CAD build for the part. Positions are in the model's coordinates, mm. Face numbers are marked on the shaded views. A direction names the side the tool comes from. Coordinates: 2 decimals unless noted, no trailing zeros. Loops run counter-clockwise (first coordinate to the right, second up) from the corner with the lowest first, then second, coordinate; pieces in that order, holes last.
1) Saw through at B-B, the plane x = 0. Write the cut outline in (y, z) (1 decimal), and give its area (3 significant figures).
2) Saw through at C-C, the plane z = 0. Write the cut outline in (x, y) (1 decimal), and give its area (3 significant figures).
3) Saw through at A-A, the plane y = -8.5. Write the cut outline in (x, z) (3 decimals), and give its area (3 significant figures).
4) Which spindle directions (+Z, -Z, +X, -X, +Y, -Y) get a long thin tool onto all of the face, cutting with end or side? Do the marked faces 4, 5 and 6. Say none if no direction does.
5) Saw through at D-D, the plane y = -16. Write the cut outline in (x, z), and give its area (3 significant figures).
6) Wall check: line 1 along Z through (x, y) = (0, -12) (3 decimals); line 2 along Z through (x, y) = (2, -12.25); line 3 along X through (y, z) = (-10.25, 2.75). Give the ranges that are in metal, low to high.
7) Pin check, flat tips, straight feed: pin 1 Ø8 at (x, y) = (5.5, -5.5) entering from +Z; pin 2 Ø1 at (y, z) = (-11.5, -4) entering from +X; pin 3 Ø3 at (x, z) = (6.5, 2) entering from -Y; pin 4 Ø9.5 at (x, z) = (-3, 2) entering from -Y. Stop position of each tip, or through.
8) Two-plate mould, pull along Z, no slides. Class the marked faces 1, 2 and 3: +Z half, -Z half, draft (parallel to the pull), parting line (faces both ways), or undercut.
```python
from build123d import *

# Parameters (mm, degrees)
F0_R     = 9.525
F1_DEPTH = 14.2875
F2_R     = 8.150668
F3_DEPTH = 1.5875
F4_R     = 7.451833
F5_DEPTH = 6.35
F6_R     = 3
F7_DEPTH = 9.525


with BuildPart() as f1:
    # F0 (on Front) → F1 (new body)
    with BuildSketch(Plane.XZ):
        Circle(F0_R)
    extrude(amount=F1_DEPTH)

    # F2 (on face) → F3 (join)
    with BuildSketch(Plane(origin=(0, 0, 0), x_dir=(-1, 0, 0), z_dir=(0, 1, 0))):
        Circle(F2_R)
    extrude(amount=F3_DEPTH)

    # F4 (on face) → F5 (cut)
    with BuildSketch(Plane.XZ.offset(14.2875)):
        Circle(F4_R)
    extrude(amount=-F5_DEPTH, mode=Mode.SUBTRACT)

    # F6 (on face) → F7 (join)
    with BuildSketch(Plane.XZ.offset(7.9375)):
        Circle(F6_R)
    extrude(amount=F7_DEPTH)


solid = f1.part
```
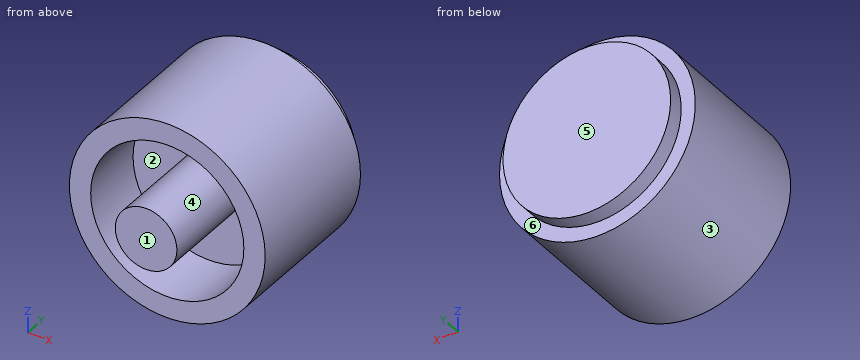
Data:
1. outline: (-17.5, -3) - (-7.9, -3) - (-7.9, -7.5) - (-14.3, -7.5) - (-14.3, -9.5) - (0, -9.5) - (0, -8.2) - (1.6, -8.2) - (1.6, 8.2) - (0, 8.2) - (0, 9.5) - (-14.3, 9.5) - (-14.3, 7.5) - (-7.9, 7.5) - (-7.9, 3) - (-17.5, 3) - close
1. area: 261 mm2
2. outline: (-9.5, -14.3) - (-7.5, -14.3) - (-7.5, -7.9) - (-3, -7.9) - (-3, -17.5) - (3, -17.5) - (3, -7.9) - (7.5, -7.9) - (7.5, -14.3) - (9.5, -14.3) - (9.5, 0) - (8.2, 0) - (8.2, 1.6) - (-8.2, 1.6) - (-8.2, 0) - (-9.5, 0) - close
2. area: 261 mm2
3. outline: circle Ø19.05 at (0, 0); circle Ø6 at (0, 0); hole circle Ø14.904 at (0, 0)
3. area: 139 mm2
4. face 4: -Y
4. face 5: +Z, -Z, +X, -X, +Y
4. face 6: +Y
5. outline: circle Ø6 at (0, 0)
5. area: 28.3 mm2
6. line 1: z = -9.525 to -7.452, -3 to 3, 7.452 to 9.525
6. line 2: z = -9.31 to -7.18, -2.24 to 2.24, 7.18 to 9.31
6. line 3: x = -9.12 to -6.93, -1.2 to 1.2, 6.93 to 9.12
7. pin 1: stops at z = 9.41
7. pin 2: stops at x = 8.86
7. pin 3: stops at y = -14.29
7. pin 4: stops at y = -17.46
8. face 1: draft
8. face 2: undercut
8. face 3: parting line
